Could you check a few things on this drawing? It's one solid part, dimensions in mm from its lowest x, y, z. A direction names the side the tool comes from. Give positions to 0.01 mm unless a question says otherwise; leave off trailing zeros. Loops run counter-clockwise (first coordinate to the right, second up) from the corner with the lowest first, then second, coordinate; pieces in that order, holes last. Notation, with made-up numbers: (10, 64) - (50, 64) arc R20 cw to (50, 71) - close; hole circle Ø8 at (-25.5, 69). An arc over 180 degrees is marked (long way). Return JSON: item names as keys, results as strings. Group by question number.
(1) I need wall thicknesses on probe 1 along Y at (x, z) = (2.75, 55); probe 2 along X at (y, z) = (63, 50); probe 3 along X at (y, z) = (19.5, 80.5). Which ranges of each line are inside material? Lowest first, please. Write a range as [from, to].
(2) If we section it at A-A (y = 55): Please give me the cut outline in (x, z).
(3) If we mould it in two halves opening along Y, with no side actions, what happens to the marked faces 1, 2 and 3? For each: released by +Y, released by -Y, zero draft, split by the parting line, or undercut.
(4) If we section it at B-B (x = 16.75): Please give me the cut outline in (y, z).
(5) For P1, Ø11, axis at y = 55, z = 55, coming from the -X side; P2, Ø10, axis at x = 6.5, z = 49.5, coming from the +Y side; P3, Ø10, axis at x = 10, z = 49.5, coming from the -Y side, each with a flat end and sliding along its axis, tell me the tip position at first contact or that it passes through.
(6) If we section it at D-D (z = 72.5): Please give me the cut outline in (x, y).
(7) On a 3-axis mill with a long thin cutter (end or side, diameter ignored), from which of +Z, -Z, +X, -X, +Y, -Y can I reach the whole of each face in a straight line? I mean the marked faces 4 and 5. Say none if no direction works.
(8) If we section it at C-C (z = 22.5): Please give me the cut outline in (x, y), then the cut area to 3 significant figures.
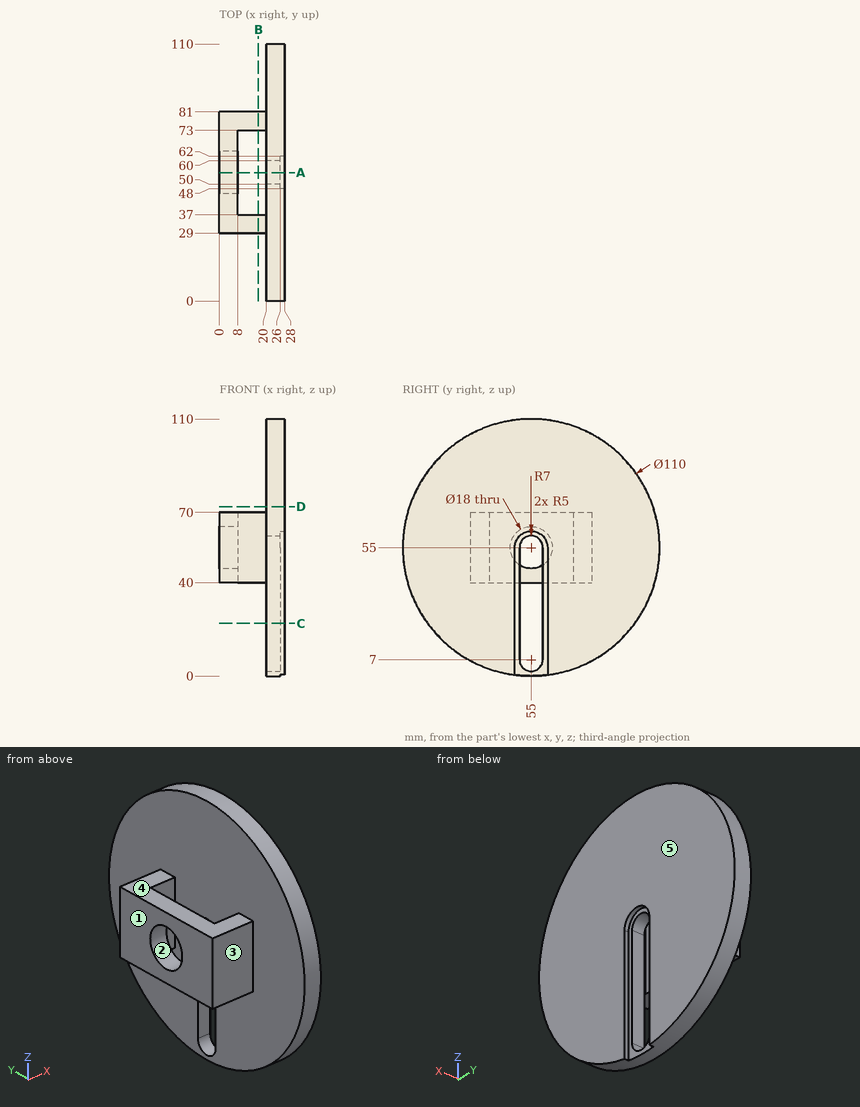
Values:
{
 "1": {"probe 1": "[29, 46], [64, 81]", "probe 2": "[0, 8], [20, 28]", "probe 3": "[20, 28]"},
 "2": {"outline": "(0, 40) - (8, 40) - (8, 46) - (0, 46) - close; (0, 64) - (8, 64) - (8, 70) - (0, 70) - close; (20, 0) - (26, 0) - (26, 2) - (20, 2) - close; (20, 60) - (26, 60) - (26, 62) - (28, 62) - (28, 110) - (20, 110) - close"},
 "3": {"face 1": "zero draft", "face 2": "undercut", "face 3": "released by -Y"},
 "4": {"outline": "(29, 40) - (37, 40) - (37, 70) - (29, 70) - close; (73, 40) - (81, 40) - (81, 70) - (73, 70) - close"},
 "5": {"P1": "x = 20", "P2": "y = 81", "P3": "y = 29"},
 "6": {"outline": "(20, 2.86) - (28, 2.86) - (28, 107.14) - (20, 107.14) - close"},
 "7": {"face 4": "+Z, -X, +Y, -Y", "face 5": "+Z, -Z, +X, +Y, -Y"},
 "8": {"outline": "(20, 10.63) - (28, 10.63) - (28, 48) - (26, 48) - (26, 50) - (20, 50) - close; (20, 60) - (26, 60) - (26, 62) - (28, 62) - (28, 99.37) - (20, 99.37) - close", "area": "622 mm2"}
}
